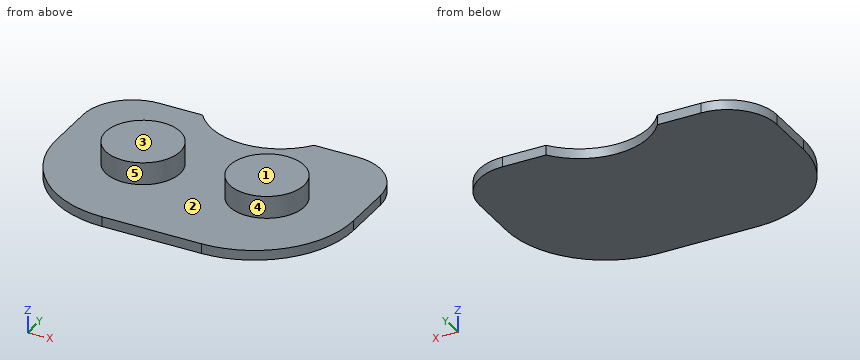
```python
from build123d import *

# Parameters (mm, degrees)
EXTRUDE_1_DEPTH = 2
SKETCH_3_R      = 7.5
EXTRUDE_2_DEPTH = 6.5


with BuildPart() as part:
    # 草图1 → 凸台-拉伸1 (new body)
    with BuildSketch(Plane.XY):
        with BuildLine():
            Line((-10, -20), (10, -20))
            ThreePointArc((10, -20), (24.142135624, -14.142135624), (30, 0))
            Line((30, 0), (30, 10))
            ThreePointArc((30, 10), (27.071067812, 17.071067812), (20, 20))
            Line((20, 20), (11.249888888, 20))
            ThreePointArc((11.249888888, 20), (0, 14.4), (-11.249888888, 20))
            Line((-11.249888888, 20), (-20, 20))
            ThreePointArc((-20, 20), (-27.071067812, 17.071067812), (-30, 10))
            Line((-30, 10), (-30, 0))
            ThreePointArc((-30, 0), (-24.142135624, -14.142135624), (-10, -20))
        make_face()
    extrude(amount=EXTRUDE_1_DEPTH)

    # 草图3 → 凸台-拉伸2 (add)
    with BuildSketch(Plane.XY):
        with Locations(Location((-12.5, 0, 0), (0, 0, 180))):
            Circle(SKETCH_3_R)
        with Locations(Location((12.5, 0, 0), (0, 0, 180))):
            Circle(SKETCH_3_R)
    extrude(amount=EXTRUDE_2_DEPTH)


solid = part.part
```
The listing builds one solid part. Answer for the finished solid, in the listing's coordinates (mm). Face numbers are marked on the shaded views. A direction names the side the tool comes from. Give positions to 0.01 mm unless a question says otherwise; leave off trailing zeros. Order: outer loops, then holes, each group sorted by start corner. A loop starts at its lowest first (then second) coordinate and runs counter-clockwise, first axis right, second up. Notation, with made-up numbers: (42.25, 14) -> (91.25, 14) arc R6 cw to (91.25, 23) -> close; hole circle Ø10 at (17, 85.25). An arc over 180 degrees is marked (long way). Write each question's results on one line, items separated by ' | '.
Q1. Each of these flat-tipped pins is pushed along its axis until it touches: P1, Ø1.5, axis at x = -10, z = 5.5, coming from the +Y side; P2, Ø1.5, axis at x = -1.5, y = 8, coming from the -Z side. Where does it stop, or does it pass through?
Checked values:
P1: stops at y = 7.29 | P2: stops at z = 0
Q2. Determine the mould class of the marked faces 3, 4 and 5 for opening direction X: pulls with the +X half, pulls with the -X half, needs draft (parallel to the pull), parting line crosses it, or undercut.
Checked values:
face 3: needs draft | face 4: undercut | face 5: undercut
Q3. The part is cut by section C-C, the plane z = 4.25. Give the vertices of the cut face in (x, y).
Checked values:
outline: circle Ø15 at (-12.5, 0); circle Ø15 at (12.5, 0)
Q4. Straight lines are drawn through the part: probe 1 along Z at (x, y) = (27, -1.5); probe 2 along X at (y, z) = (-5.5, 2.75); probe 3 along X at (y, z) = (-3, 3). For each, find the intervals that lie inside material, in ascending order. Write a range as from..to.
Checked values:
probe 1: z = 0..2 | probe 2: x = -17.6..-7.4, 7.4..17.6 | probe 3: x = -19.37..-5.63, 5.63..19.37
Q5. Which of the six approach directions +Z, -Z, +X, -X, +Y, -Y give full straight-line access (tool end or side, diameter ignored) to the marked faces 1 and 2?
Checked values:
face 1: +Z, +X, -X, +Y, -Y | face 2: +Z
Q6. The part is cut by section D-D, the plane x = 12.5. Give the vertices of the cut face in (y, z), and give its area (3 significant figures).
Checked values:
outline: (-19.84, 0) -> (20, 0) -> (20, 2) -> (7.5, 2) -> (7.5, 6.5) -> (-7.5, 6.5) -> (-7.5, 2) -> (-19.84, 2) -> close | area: 147 mm^2
Q7. The part is cut by section A-A, the plane z = 1.25. Give the vertices of the cut face in (x, y), and give its area (3 significant figures).
Checked values:
outline: (-30, 0) arc R20 ccw to (-10, -20) -> (10, -20) arc R20 ccw to (30, 0) -> (30, 10) arc R10 ccw to (20, 20) -> (11.25, 20) arc R14.1 cw to (-11.25, 20) -> (-20, 20) arc R10 ccw to (-30, 10) -> close | area: 2,100 mm^2
Q8. The part is cut by section B-B, the plane y = 17.5. Give the vertices of the cut face in (x, z).
Checked values:
outline: (-26.61, 0) -> (-8.82, 0) -> (-8.82, 2) -> (-26.61, 2) -> close; (8.82, 0) -> (26.61, 0) -> (26.61, 2) -> (8.82, 2) -> close
